```python
from build123d import *

# Parameters (mm, degrees)
F1_D     = 7.5
F6_DEPTH = 56.015512
F7_R     = 46
F7_R_2   = 3.75
F2_DEPTH = 10


with BuildPart() as f5:
    # F4 (on Front) → F5 (revolve)
    with BuildSketch(Plane.XZ):
        with BuildLine():
            Line((0, 4.45), (0, -14.164552))
            Line((0, -14.164552), (48.5, -14.164552))
            ThreePointArc((48.5, -14.164552), (48.853553, -14.018106), (49, -13.664552))
            ThreePointArc((49, -13.664552), (48.949039, -13.419799), (48.900011, -13.174652))
            ThreePointArc((48.900011, -13.174652), (48.630694, -12.543302), (48.670812, -11.858083))
            ThreePointArc((48.670812, -11.858083), (48.633742, -11.608227), (48.598665, -11.358083))
            ThreePointArc((48.598665, -11.358083), (48.366471, -10.712157), (48.446319, -10.030424))
            ThreePointArc((48.446319, -10.030424), (48.322268, -6.161579), (48.670812, -2.306469))
            ThreePointArc((48.670812, -2.306469), (48.630694, -1.62125), (48.900011, -0.9899))
            ThreePointArc((48.900011, -0.9899), (48.949039, -0.744753), (49, -0.5))
            ThreePointArc((49, -0.5), (48.853553, -0.146447), (48.5, 0))
            Line((48.5, 0), (41, 0))
            Line((41, 0), (41, 4.45))
            Line((41, 4.45), (0, 4.45))
        make_face()
    revolve(axis=Axis((0, 0, -4.857276), (0, 0, -1)))

    # F1 (through all)
    with Locations(Plane.XY.offset(4.45)):
        with Locations((0, 0)):
            Hole(F1_D / 2)

    # F0 (on face) → F6 (cut)
    with BuildSketch(Plane.XY.offset(4.45)):
        with BuildLine():
            ThreePointArc((-3.75, 28.695601), (-5.774405, 32.713789), (-10.208333, 33.478201))
            ThreePointArc((-10.208333, 33.478201), (-24.748737, 24.748737), (-33.478201, 10.208333))
            ThreePointArc((-33.478201, 10.208333), (-32.713789, 5.774405), (-28.695601, 3.75))
            Line((-28.695601, 3.75), (-6.495191, 3.75))
            ThreePointArc((-6.495191, 3.75), (-5.303301, 5.303301), (-3.75, 6.495191))
            Line((-3.75, 6.495191), (-3.75, 28.695601))
        make_face()
        with BuildLine():
            Line((-3.75, -28.695601), (-3.75, -6.495191))
            ThreePointArc((-3.75, -6.495191), (-5.303301, -5.303301), (-6.495191, -3.75))
            Line((-6.495191, -3.75), (-28.695601, -3.75))
            ThreePointArc((-28.695601, -3.75), (-32.713789, -5.774405), (-33.478201, -10.208333))
            ThreePointArc((-33.478201, -10.208333), (-24.748737, -24.748737), (-10.208333, -33.478201))
            ThreePointArc((-10.208333, -33.478201), (-5.774405, -32.713789), (-3.75, -28.695601))
        make_face()
        with BuildLine():
            ThreePointArc((33.478201, -10.208333), (32.713789, -5.774405), (28.695601, -3.75))
            Line((28.695601, -3.75), (6.495191, -3.75))
            ThreePointArc((6.495191, -3.75), (5.303301, -5.303301), (3.75, -6.495191))
            Line((3.75, -6.495191), (3.75, -28.695601))
            ThreePointArc((3.75, -28.695601), (5.774405, -32.713789), (10.208333, -33.478201))
            ThreePointArc((10.208333, -33.478201), (24.748737, -24.748737), (33.478201, -10.208333))
        make_face()
        with BuildLine():
            ThreePointArc((10.208333, 33.478201), (5.774405, 32.713789), (3.75, 28.695601))
            Line((3.75, 28.695601), (3.75, 6.495191))
            ThreePointArc((3.75, 6.495191), (5.303301, 5.303301), (6.495191, 3.75))
            Line((6.495191, 3.75), (28.695601, 3.75))
            ThreePointArc((28.695601, 3.75), (32.713789, 5.774405), (33.478201, 10.208333))
            ThreePointArc((33.478201, 10.208333), (24.748737, 24.748737), (10.208333, 33.478201))
        make_face()
    extrude(amount=-F6_DEPTH, mode=Mode.SUBTRACT)

    # F7 (on face) → F2 (cut)
    with BuildSketch(Plane(origin=(0, 0, -14.164552), x_dir=(1, 0, 0), z_dir=(0, 0, -1))):
        Circle(F7_R)
        with BuildLine():
            ThreePointArc((-6.495191, -3.75), (-5.303301, -5.303301), (-3.75, -6.495191))
            Line((-3.75, -6.495191), (-3.75, -28.695601))
            ThreePointArc((-3.75, -28.695601), (-5.774405, -32.713789), (-10.208333, -33.478201))
            ThreePointArc((-10.208333, -33.478201), (-24.748737, -24.748737), (-33.478201, -10.208333))
            ThreePointArc((-33.478201, -10.208333), (-32.713789, -5.774405), (-28.695601, -3.75))
            Line((-28.695601, -3.75), (-6.495191, -3.75))
        make_face(mode=Mode.SUBTRACT)
        with BuildLine():
            ThreePointArc((33.478201, -10.208333), (24.748737, -24.748737), (10.208333, -33.478201))
            ThreePointArc((10.208333, -33.478201), (5.774405, -32.713789), (3.75, -28.695601))
            Line((3.75, -28.695601), (3.75, -6.495191))
            ThreePointArc((3.75, -6.495191), (5.303301, -5.303301), (6.495191, -3.75))
            Line((6.495191, -3.75), (28.695601, -3.75))
            ThreePointArc((28.695601, -3.75), (32.713789, -5.774405), (33.478201, -10.208333))
        make_face(mode=Mode.SUBTRACT)
        with BuildLine():
            ThreePointArc((-33.478201, 10.208333), (-24.748737, 24.748737), (-10.208333, 33.478201))
            ThreePointArc((-10.208333, 33.478201), (-5.774405, 32.713789), (-3.75, 28.695601))
            Line((-3.75, 28.695601), (-3.75, 6.495191))
            ThreePointArc((-3.75, 6.495191), (-5.303301, 5.303301), (-6.495191, 3.75))
            Line((-6.495191, 3.75), (-28.695601, 3.75))
            ThreePointArc((-28.695601, 3.75), (-32.713789, 5.774405), (-33.478201, 10.208333))
        make_face(mode=Mode.SUBTRACT)
        Circle(F7_R_2, mode=Mode.SUBTRACT)
        with BuildLine():
            ThreePointArc((10.208333, 33.478201), (24.748737, 24.748737), (33.478201, 10.208333))
            ThreePointArc((33.478201, 10.208333), (32.713789, 5.774405), (28.695601, 3.75))
            Line((28.695601, 3.75), (6.495191, 3.75))
            ThreePointArc((6.495191, 3.75), (5.303301, 5.303301), (3.75, 6.495191))
            Line((3.75, 6.495191), (3.75, 28.695601))
            ThreePointArc((3.75, 28.695601), (5.774405, 32.713789), (10.208333, 33.478201))
        make_face(mode=Mode.SUBTRACT)
    extrude(amount=-F2_DEPTH, mode=Mode.SUBTRACT)


solid = f5.part
```
Geometry check sheet. Reference: the model listing, model coordinates, mm. A direction names the side the tool comes from. Coordinates: 2 decimals unless noted, no trailing zeros. Loops run counter-clockwise (first coordinate to the right, second up) from the corner with the lowest first, then second, coordinate; pieces in that order, holes last. Notation, with made-up numbers: (-31.75, 64.5) - (1.25, 64.5) arc R11 ccw to (1.25, 68.5) - close; hole circle Ø8 at (-35.5, 76). An arc over 180 degrees is marked (long way). One line per item, written item: value. Start each with the question number.
(1) Depth check by flat-ended pin: P1, Ø4.5, axis at y = 14, z = 1, coming from the -X side; P2, Ø2.5, axis at x = -20.5, z = 0, coming from the +Y side; P3, Ø1.5, axis at y = -27, z = -8.5, coming from the +X side; P4, Ø3, axis at x = 15, y = 29.5, coming from the -Z side. Enter the tip coordinate at first touch or a pass-through.
(2) Cross-section at D-D on z = -7.5. Enter the section's corners in (x, y), plus the area to 3 significant figures.
(3) Cross-section at C-C on y = -24. Count the separate pieces of the cut face and the enclosed holes in it, plus the area to 3 significant figures.
(4) Material ranges on line 1 (X direction, y = 29, z = -2.75); line 2 (Y direction, x = 0, z = 1); line 3 (Z direction, x = -26, y = 28), recorded low to high. Write a range as [from, to].
(5) Cross-section at B-B on z = 2.75. Enter the section's corners in (x, y), plus the area to 3 significant figures.
(6) Tool access check on faces 3 (the cylindrical face through (-5.99, -45.61, -9.23)), 4 (the flat face through (-18, 3.75, 0)). Record the directions out of +Z, -Z, +X, -X, +Y, -Y that give a thin tool (end or side, any length) a straight path to the whole face; none if there is none.
(7) Mould release check, pull along X, two halves, no side actions. Record for faces 1 (the flat face through (-1, 10, -4.165)), 2 (the cylindrical face through (-9, 40, 2)): released by +X, released by -X, zero draft, split by the parting line, or undercut.
Results below:
1. P1: stops at x = -47.44
1. P2: stops at y = 45.02
1. P3: stops at x = 40.59
1. P4: passes through
2. outline: circle Ø96.62 at (0, 0); hole circle Ø92 at (0, 0)
2. area: 685 mm2
3. separate pieces: 3
3. enclosed holes: 0
3. area: 332 mm2
4. line 1: x = [-39.01, -19.6], [-3.76, 3.76], [19.6, 39.01]
4. line 2: y = [-41, -3.75], [3.75, 41]
4. line 3: z = [-4.16, 4.45]
5. outline: circle Ø82 at (0, 0); hole (-33.48, -10.21) arc R35 ccw to (-10.21, -33.48) arc R5 ccw to (-3.75, -28.7) - (-3.75, -6.5) arc R7.5 cw to (-6.5, -3.75) - (-28.7, -3.75) arc R5 ccw to start; hole (-33.48, 10.21) arc R5 ccw to (-28.7, 3.75) - (-6.5, 3.75) arc R7.5 cw to (-3.75, 6.5) - (-3.75, 28.7) arc R5 ccw to (-10.21, 33.48) arc R35 ccw to start; hole circle Ø7.5 at (0, 0); hole (3.75, -28.7) arc R5 ccw to (10.21, -33.48) arc R35 ccw to (33.48, -10.21) arc R5 ccw to (28.7, -3.75) - (6.5, -3.75) arc R7.5 cw to (3.75, -6.5) - close; hole (3.75, 6.5) arc R7.5 cw to (6.5, 3.75) - (28.7, 3.75) arc R5 ccw to (33.48, 10.21) arc R35 ccw to (10.21, 33.48) arc R5 ccw to (3.75, 28.7) - close
5. area: 2,470 mm2
6. face 3: -Z
6. face 4: +Z, -Z
7. face 1: undercut
7. face 2: split by the parting line
